Model file for the job. Use its own axes, mm. Face numbers are marked on the shaded views. Round coordinates to 2 decimals unless told otherwise and drop trailing zeros. Order: outer loops, then holes, each group sorted by start corner. A loop starts at its lowest first (then second) coordinate and runs counter-clockwise, first axis right, second up. Notation, with made-up numbers: (-35, -25.75) - (7, -25.75) arc R20 cw to (7, 2.25) - close; hole circle Ø6 at (-3, 31). An arc over 180 degrees is marked (long way). Put each result on its own line as item: value. Start each with the question number.
Item 1: Saw through at A-A on y = 0. List the corners of the cut face in (x, z).
Item 2: Saw through at D-D on z = 17.5. List the corners of the cut face in (x, y).
Item 3: Pin check, flat tips, straight feed: pin 1 Ø2 at (x, z) = (-2.5, 4.5) entering from -Y; pin 2 Ø2 at (x, z) = (3.5, 17) entering from +Y. Stop position of each tip, or through.
Item 4: Saw through at C-C on z = 11.5. List the corners of the cut face in (x, y).
Item 5: Probe probe 1 along X at (y, z) = (0, 12); probe 2 along Z at (x, y) = (-0.5, 1.75); probe 3 along Y at (x, z) = (-0.25, 9.25). List the from-to ranges inside material, lowest first.
Item 6: Mould opens along Y. For the marked faces 1, 2 and 3 say: pulls with the +Y half, pulls with the -Y half, needs draft (parallel to the pull), parting line crosses it, or undercut.
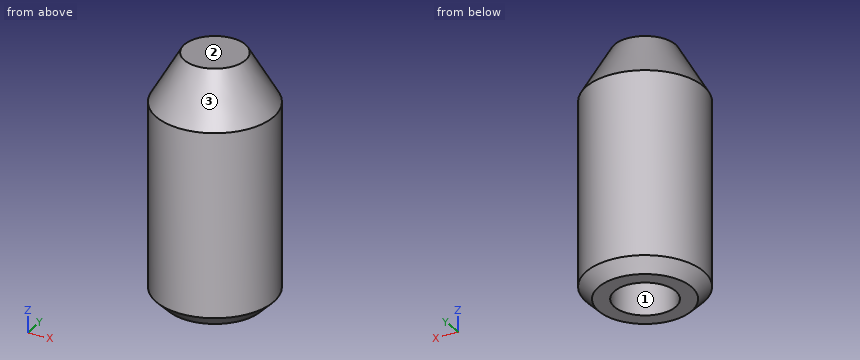
```python
from build123d import *

# Parameters (mm, degrees)
F2_SIZE  = 1
F3_SIZE2 = 2.309401
F3_SIZE  = 4


with BuildPart() as f1:
    # F0 (on Right) → F1 (revolve)
    with BuildSketch(Plane.YZ):
        Polygon((2.5, 17), (2.5, 0), (4.8, 0), (4.8, 20), (0, 20), (0, 17), align=None)
    revolve(axis=Axis((0, 0, 15.318091), (0, 0, -1)))

    # F2
    f2_edges = [f1.edges().sort_by_distance(p)[0] for p in [
        (0, -4.8, 0),
    ]]
    chamfer(f2_edges, length=F2_SIZE)

    # F3
    f3_edges = [f1.edges().sort_by_distance(p)[0] for p in [
        (0, -4.8, 20),
    ]]
    chamfer(f3_edges, length=F3_SIZE, length2=F3_SIZE2)


solid = f1.part
```
Results found:
1. outline: (-4.8, 1) - (-3.8, 0) - (-2.5, 0) - (-2.5, 17) - (2.5, 17) - (2.5, 0) - (3.8, 0) - (4.8, 1) - (4.8, 16) - (2.49, 20) - (-2.49, 20) - (-4.8, 16) - close
2. outline: circle Ø7.87 at (0, 0)
3. pin 1: stops at y = -4.56
3. pin 2: stops at y = 3.69
4. outline: circle Ø9.6 at (0, 0); hole circle Ø5 at (0, 0)
5. probe 1: x = -4.8 to -2.5, 2.5 to 4.8
5. probe 2: z = 17 to 20
5. probe 3: y = -4.79 to -2.49, 2.49 to 4.79
6. face 1: undercut
6. face 2: needs draft
6. face 3: parting line crosses it
